from build123d import *


with BuildPart() as part:
    # Sketch1 → Revolve1 (revolve)
    with BuildSketch(Plane.XY):
        with BuildLine():
            Line((19, 34.18946336), (19, -10.81053664))
            Line((19, -10.81053664), (25, -10.81053664))
            Line((25, -10.81053664), (25, 14.18946336))
            Line((25, 14.18946336), (40, 14.18946336))
            ThreePointArc((40, 14.18946336), (45.084745763, 19.274209123), (40, 24.358954886))
            Line((40, 24.358954886), (40, 24.18946336))
            Line((40, 24.18946336), (25, 24.18946336))
            Line((25, 24.18946336), (25, 34.18946336))
            Line((25, 34.18946336), (19, 34.18946336))
        make_face()
    revolve(axis=Axis((0, 56.797792619, 0), (0, -1, 0)))


solid = part.part
Verification items for the finished model (mm, model axes). A direction names the side the tool comes from. Coordinates: 2 decimals unless noted, no trailing zeros. Order: outer loops, then holes, each group sorted by start corner. A loop starts at its lowest first (then second) coordinate and runs counter-clockwise, first axis right, second up.
Item 1: Section check B-B, the plane x = 0. Enter the section's corners in (y, z), then the cut area to 3 significant figures.
Filled in:
outline: (-10.81, -25) - (14.19, -25) - (14.19, -40) arc R5.08 ccw to (24.36, -40) - (24.19, -40) - (24.19, -25) - (34.19, -25) - (34.19, -19) - (-10.81, -19) - close; (-10.81, 19) - (34.19, 19) - (34.19, 25) - (24.19, 25) - (24.19, 40) - (24.36, 40) arc R5.08 ccw to (14.19, 40) - (14.19, 25) - (-10.81, 25) - close
area: 921 mm2
Item 2: Section check A-A, the plane z = 0. Enter the section's corners in (x, y).
Filled in:
outline: (-40, 14.19) - (-25, 14.19) - (-25, -10.81) - (-19, -10.81) - (-19, 34.19) - (-25, 34.19) - (-25, 24.19) - (-40, 24.19) - (-40, 24.36) arc R5.08 ccw to start; (19, -10.81) - (25, -10.81) - (25, 14.19) - (40, 14.19) arc R5.08 ccw to (40, 24.36) - (40, 24.19) - (25, 24.19) - (25, 34.19) - (19, 34.19) - close
Item 3: Depth check by flat-ended pin: pin 1 (6 mm diameter, centred on y = 16, z = 25.5, fed in from -X); pin 2 (1 mm diameter, centred on x = -12.5, z = 14, fed in from +Y); pin 3 (2 mm diameter, centred on x = -34, y = 20, fed in from -Z); pin 4 (8 mm diameter, centred on x = 35.5, y = 29.5, fed in from -Z). Enter the tip coordinate at first touch or a pass-through.
Filled in:
pin 1: stops at x = -38.47
pin 2: stops at y = 34.19
pin 3: stops at z = -30.66
pin 4: passes through
Item 4: Release check for a two-part mould opening along Z. For faces 1 (the face through (23.846, 1.864, 7.509)), 2 (the face through (17.22, 24.189, 18.34)), 3 (the face through (4, -10.811, 19)) record: +Z half, -Z half, draft (parallel to the pull), parting line (faces both ways), or undercut.
Filled in:
face 1: parting line
face 2: undercut
face 3: draft
Item 5: Material ranges on L1, parallel to Z at x = 0, y = 19.5; L2, parallel to Z at x = 0, y = 4; L3, parallel to Y at x = 13.5, z = 38, recorded low to high.
Filled in:
L1: z = -45.08 to -19, 19 to 45.08
L2: z = -25 to -19, 19 to 25
L3: y = 14.2 to 24.35
Item 6: Access from +Z, -Z, +X, -X, +Y, -Y to the whole of each face (thin tool, end or side, straight path). Record for faces 4 (the face through (-17.22, 14.189, 18.34)), 5 (the face through (23.846, 29.259, 7.509)), 6 (the face through (-4, 34.189, 19)).
Filled in:
face 4: -Y
face 5: +Y
face 6: +Z, -Z, +X, -X, +Y
Item 7: Section check C-C, the plane y = 22.5. Enter the section's corners in (x, z), then the cut area to 3 significant figures.
Filled in:
outline: circle Ø87.86 at (0, 0); hole circle Ø38 at (0, 0)
area: 4,930 mm2
